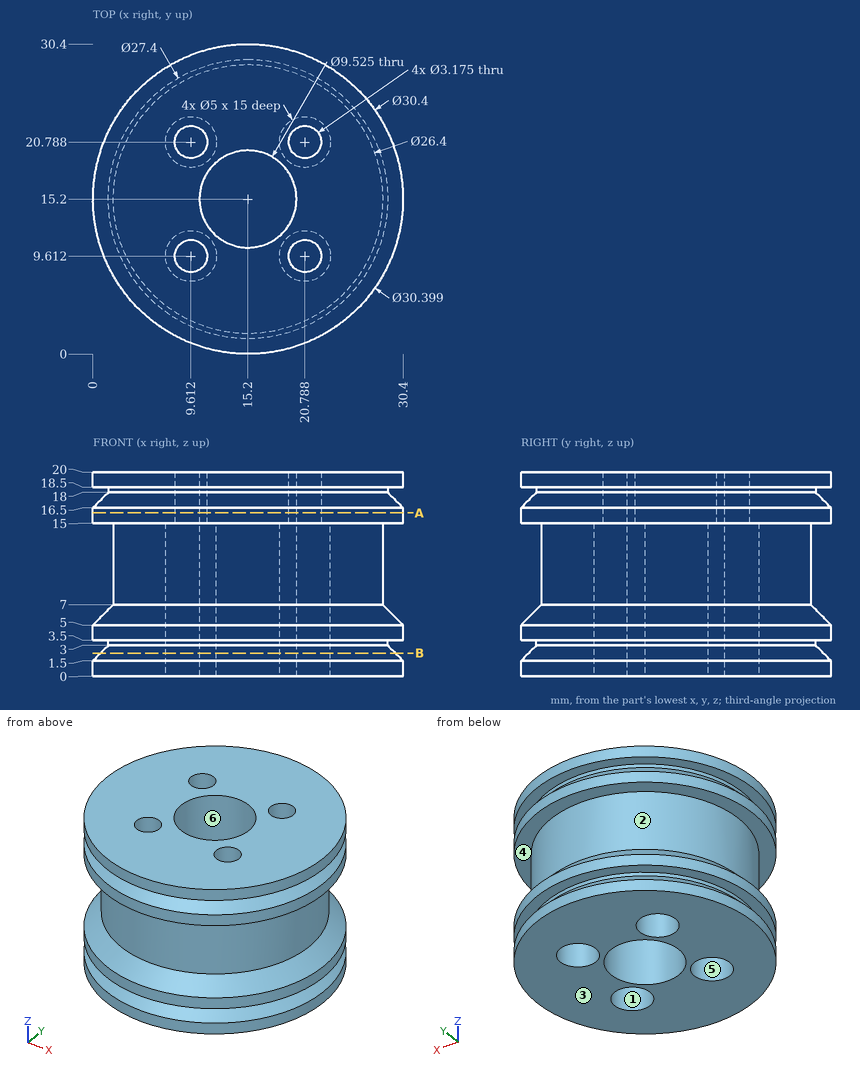
Drawing for the job (mm, zero at the part's lowest x, y, z). A direction names the side the tool comes from. Give positions to 0.01 mm unless a question says otherwise; leave off trailing zeros. Write each loop counter-clockwise with the first axis right and the second up, starting at its lowest first coordinate (ties: lowest second). Pieces come first, ordered by that corner, then holes. Notation, with made-up numbers: (9, 34.25) - (62, 34.25) arc R19 ccw to (62, 58.25) - close; hole circle Ø10 at (42, 44). An arc over 180 degrees is marked (long way). Answer as CSV lines item,"result".
Q1. Flat gauge pins, fed straight in: pin 1 Ø6 at (y, z) = (10, 14.5) entering from -X; pin 2 Ø5.5 at (x, y) = (9.5, 21.5) entering from -Z; pin 3 Ø3 at (x, z) = (8.5, 9) entering from -Y; pin 4 Ø4 at (y, z) = (24.5, 8) entering from -X. Where does each tip first touch, or does it go through?
Result set:
pin 1,"x = 0.17"
pin 2,"z = 0"
pin 3,"y = 3.07"
pin 4,"x = 4.01"
Q2. Band-saw the part on B-B (z = 2.25). State how many separate pieces and enclosed holes the cut face has, and give its area (3 significant figures).
Result set:
separate pieces,"1"
enclosed holes,"5"
area,"506 mm²"
Q3. 3-axis set-ups, long thin cutter, end or side, ignore diameter. For the marked faces 4, 5 and 6: which of +Z, -Z, +X, -X, +Y, -Y reach the whole face in a straight line?
Result set:
face 4,"none"
face 5,"-Z"
face 6,"+Z, -Z"
Q4. Band-saw the part on A-A (z = 16). Give the cut face in (x, y) (1 decimal).
Result set:
outline,"circle Ø30.4 at (15.2, 15.2); hole circle Ø3.2 at (9.6, 9.6); hole circle Ø3.2 at (9.6, 20.8); hole circle Ø9.5 at (15.2, 15.2); hole circle Ø3.2 at (20.8, 9.6); hole circle Ø3.2 at (20.8, 20.8)"
Q5. Drill centre lines: line 1 (X direction, y = 15.2, z = 14.25); line 2 (X direction, y = 20, z = 19.25) (1 decimal); line 3 (Y direction, x = 22.5, z = 4.5) (1 decimal). Where is each one in solid material? Low to high. Write a range as from..to.
Result set:
line 1,"2..10.44, 19.96..28.4"
line 2,"0.8..8.2, 11..19.4, 22.2..29.6"
line 3,"1.9..7.8, 11.4..19, 22.6..28.5"
Q6. Pull direction X, two halves, no side cores. Call the marked faces 1, 2 and 3: released by +X, released by -X, zero draft, split by the parting line, or undercut.
Result set:
face 1,"undercut"
face 2,"split by the parting line"
face 3,"zero draft"
